Geometry: final body of the model. Coordinates: model frame, mm. Give positions to 0.01 mm unless a question says otherwise; leave off trailing zeros. Write each loop counter-clockwise with the first axis right and the second up, starting at its lowest first coordinate (ties: lowest second). Pieces come first, ordered by that corner, then holes.
from build123d import *

# Parameters (mm, degrees)
SKETCH_1_R          = 2
SKETCH_1_R_2        = 2.08
SKETCH_1_R_3        = 5
SKETCH_1_R_4        = 3
EXTRUDE_1_DEPTH     = 2
CUT_EXTRUDE_1_DEPTH = 1


with BuildPart() as part:
    # 草图1 → 凸台-拉伸1 (new body)
    with BuildSketch(Plane.XY):
        with BuildLine():
            Line((26.233844386, -52.574512395), (29.233844386, -52.574512395))
            Line((29.233844386, -52.574512395), (29.233844386, -47.574512395))
            Line((29.233844386, -47.574512395), (26.233844386, -47.574512395))
            Line((26.233844386, -47.574512395), (26.233844386, -12.754512395))
            Line((26.233844386, -12.754512395), (29.233844386, -12.754512395))
            Line((29.233844386, -12.754512395), (29.233844386, -4.754512395))
            Line((29.233844386, -4.754512395), (26.233844386, -4.754512395))
            Line((26.233844386, -4.754512395), (26.233844386, -4.654512395))
            Line((26.233844386, -4.654512395), (26.233844386, 12.425487605))
            Line((26.233844386, 12.425487605), (16.233844386, 22.425487605))
            Line((16.233844386, 22.425487605), (12.733844386, 22.425487605))
            ThreePointArc((12.733844386, 22.425487605), (-2.266155614, 37.425487605), (-17.266155614, 22.425487605))
            Line((-17.266155614, 22.425487605), (-20.766155614, 22.425487605))
            Line((-20.766155614, 22.425487605), (-30.766155614, 12.425487605))
            Line((-30.766155614, 12.425487605), (-30.766155614, -4.654512395))
            Line((-30.766155614, -4.654512395), (-30.766155614, -4.754512395))
            Line((-30.766155614, -4.754512395), (-33.766155614, -4.754512395))
            Line((-33.766155614, -4.754512395), (-33.766155614, -12.754512395))
            Line((-33.766155614, -12.754512395), (-30.766155614, -12.754512395))
            Line((-30.766155614, -12.754512395), (-30.766155614, -47.574512395))
            Line((-30.766155614, -47.574512395), (-33.766155614, -47.574512395))
            Line((-33.766155614, -47.574512395), (-33.766155614, -52.574512395))
            Line((-33.766155614, -52.574512395), (-30.766155614, -52.574512395))
            Line((-30.766155614, -52.574512395), (-30.766155614, -54.574512395))
            Line((-30.766155614, -54.574512395), (-30.766155614, -57.574512395))
            Line((-30.766155614, -57.574512395), (-30.766155614, -62.574512395))
            Line((-30.766155614, -62.574512395), (-33.766155614, -62.574512395))
            Line((-33.766155614, -62.574512395), (-33.766155614, -67.574512395))
            Line((-33.766155614, -67.574512395), (-30.766155614, -67.574512395))
            Line((-30.766155614, -67.574512395), (-30.766155614, -70.574512395))
            ThreePointArc((-30.766155614, -70.574512395), (-23.533087643, -90.212600129), (-4.532311227, -98.984273724))
            Line((-4.532311227, -98.984273724), (-2.266155614, -110.984273724))
            Line((-2.266155614, -110.984273724), (0, -98.984273724))
            ThreePointArc((0, -98.984273724), (19.000776416, -90.212600129), (26.233844386, -70.574512395))
            Line((26.233844386, -70.574512395), (26.233844386, -67.574512395))
            Line((26.233844386, -67.574512395), (29.233844386, -67.574512395))
            Line((29.233844386, -67.574512395), (29.233844386, -62.574512395))
            Line((29.233844386, -62.574512395), (26.233844386, -62.574512395))
            Line((26.233844386, -62.574512395), (26.233844386, -57.574512395))
            Line((26.233844386, -57.574512395), (26.233844386, -54.574512395))
            Line((26.233844386, -54.574512395), (26.233844386, -52.574512395))
        make_face()
        with Locations((-2.266155614, -85.571739483)):
            Circle(SKETCH_1_R, mode=Mode.SUBTRACT)
        with Locations((-15.254135258, -78.073125939)):
            Circle(SKETCH_1_R, mode=Mode.SUBTRACT)
        with Locations((-15.254135258, -63.075898852)):
            Circle(SKETCH_1_R, mode=Mode.SUBTRACT)
        with Locations((-2.266155614, -55.577285308)):
            Circle(SKETCH_1_R, mode=Mode.SUBTRACT)
        with Locations((10.721824031, -63.075898852)):
            Circle(SKETCH_1_R, mode=Mode.SUBTRACT)
        with Locations((10.721824031, -78.073125939)):
            Circle(SKETCH_1_R, mode=Mode.SUBTRACT)
        with Locations((-15.796155614, -70.574512395)):
            Circle(SKETCH_1_R_2, mode=Mode.SUBTRACT)
        with Locations((4.498844386, -58.857188682)):
            Circle(SKETCH_1_R_2, mode=Mode.SUBTRACT)
        with Locations((4.498844386, -82.291836109)):
            Circle(SKETCH_1_R_2, mode=Mode.SUBTRACT)
        with Locations((-2.266155614, -70.574512395)):
            Circle(SKETCH_1_R_3, mode=Mode.SUBTRACT)
        with Locations((-2.266155614, -12.754512395)):
            Circle(SKETCH_1_R_4, mode=Mode.SUBTRACT)
        with Locations((-2.266155614, 6.245487605)):
            Circle(SKETCH_1_R_4, mode=Mode.SUBTRACT)
        with Locations((-2.266155614, 25.245487605)):
            Circle(SKETCH_1_R_4, mode=Mode.SUBTRACT)
    extrude(amount=EXTRUDE_1_DEPTH)

    # 草图2 → 切除-拉伸1 (cut)
    with BuildSketch(Plane.XY.offset(2)):
        with BuildLine():
            Line((12.733844386, -19.749278663), (11.733844386, -19.749278663))
            ThreePointArc((11.733844386, -19.749278663), (12.733844386, -20.749278663), (13.733844386, -19.749278663))
            ThreePointArc((13.733844386, -19.749278663), (13.440951168, -19.042171882), (12.733844386, -18.749278663))
            Line((12.733844386, -18.749278663), (12.733844386, -19.749278663))
        make_face()
    extrude(amount=-CUT_EXTRUDE_1_DEPTH, mode=Mode.SUBTRACT)


solid = part.part
Q1. Section A-A on y = -3. Output: boundary loops of the cut face in (x, z), plus the area to 3 significant figures.
Filled sheet:
outline: (-30.77, 0) - (26.23, 0) - (26.23, 2) - (-30.77, 2) - close
area: 114 mm2
Q2. Ray query, line 1 along Y through (x, z) = (10, 0.25); line 2 along Y through (x, z) = (11.5, 0.55); line 3 along Y through (x, z) = (-14, 1.2). Return the intervals inside material, ascending.
Filled sheet:
line 1: y = -96.66 to -79.94, -76.21 to -64.94, -61.21 to 31.06
line 2: y = -95.94 to -79.92, -76.23 to -64.92, -61.23 to 28.38
line 3: y = -96.89 to -79.63, -76.52 to -71.62, -69.53 to -64.63, -61.52 to 31.77
Q3. Pin query (flat end, axial travel): P1, Ø1, axis at x = 28, z = 1, coming from the +Y side; P2, Ø0.6, axis at y = -55.5, z = 0.5, coming from the +X side. Return the tip coordinate at first contact, or that it passes through.
Filled sheet:
P1: stops at y = -4.75
P2: stops at x = 26.23
Q4. Section B-B on x = -9.5. Output: boundary loops of the cut face in (y, z).
Filled sheet:
outline: (-98.33, 0) - (35.57, 0) - (35.57, 2) - (-98.33, 2) - close
Q5. Pull-direction query (X, two-part tool) for faces 1 (the cylindrical face through (10.461, -61.093, 0.986)), 2 (the cylindrical face through (-1.94, 37.42, 0.99)), 3 (the flat face through (-25.696, 17.495, 0.986)); classes: released by +X, released by -X, zero draft, split by the parting line, or undercut.
Filled sheet:
face 1: undercut
face 2: split by the parting line
face 3: released by -X
Q6. Section C-C on z = 0.6. Count the separate pieces of the cut face and the enclosed holes in it, plus the area to 3 significant figures.
Filled sheet:
separate pieces: 1
enclosed holes: 13
area: 6,710 mm2
